```python
from build123d import *

# Parameters (mm, degrees)
SKETCH2_W            = 10
SKETCH2_H            = 14.768412439
BOSS_EXTRUDE1_DEPTH  = 5
BOSS_EXTRUDE4_DEPTH  = 10
SKETCH9_W            = 10
SKETCH9_H            = 3.18
SKETCH9_H_2          = 3.888412439
CUT_EXTRUDE3_DEPTH   = 5
BOSS_EXTRUDE5_DEPTH  = 7.7
SKETCH12_R           = 0.75
BOSS_EXTRUDE7_DEPTH  = 2.75
FILLET1_R            = 2.5
SKETCH13_W           = 17.887250462
SKETCH13_H           = 46.229219396
CUT_EXTRUDE4_DEPTH   = 20
SKETCH15_W           = 10
SKETCH15_H           = 7.7
BOSS_EXTRUDE9_DEPTH  = 100
CUT_EXTRUDE5_DEPTH   = 100
SKETCH17_W           = 2.538779858
SKETCH17_H           = 107.754476916
BOSS_EXTRUDE10_DEPTH = 5
FILLET2_R            = 3
FILLET3_R            = 3


with BuildPart() as part:
    # Sketch2 → Boss-Extrude1 (new body)
    with BuildSketch(Plane.XY):
        with Locations((0, 1.566049366)):
            Rectangle(SKETCH2_W, SKETCH2_H)
    extrude(amount=BOSS_EXTRUDE1_DEPTH)

    # Sketch8 → Boss-Extrude4 (add)
    with BuildSketch(Plane.ZY.offset(5)):
        Polygon((-0.15, 5.770255585), (0, 5.770255585), (0, 4.070255585), (-0.15, 4.070255585), (-2.137867966, 4.070255585), (-3.402081528, 5.334469147), (-2.2, 6.536550675), (-1.43370491, 5.770255585), align=None)
        Polygon((-0.15, -1.929744415), (0, -1.929744415), (0, -0.229744415), (-0.15, -0.229744415), (-1.43370491, -0.229744415), (-2.2, 0.536550675), (-3.402081528, -0.665530853), (-2.137867966, -1.929744415), align=None)
    extrude(amount=-BOSS_EXTRUDE4_DEPTH)

    # Sketch9 → Cut-Extrude3 (cut)
    with BuildSketch(Plane(origin=(0, 0, 0), x_dir=(-1, 0, 0), z_dir=(0, 0, -1))):
        with Locations((0, 7.360255585)):
            Rectangle(SKETCH9_W, SKETCH9_H)
        with Locations((0, -3.873950635)):
            Rectangle(SKETCH9_W, SKETCH9_H_2)
    extrude(amount=-CUT_EXTRUDE3_DEPTH, mode=Mode.SUBTRACT)

    # Sketch10 → Boss-Extrude5 (add)
    with BuildSketch(Plane(origin=(0, 5.770255585, 0), x_dir=(1, 0, 0), z_dir=(0, 1, 0))):
        with BuildLine():
            Line((-5, -5), (-5, -10.5))
            Line((-5, -10.5), (1.352445729, -55.7))
            Line((1.352445729, -55.7), (6.352445729, -55.7))
            Line((6.352445729, -55.7), (6.352445729, -49.2))
            ThreePointArc((6.352445729, -49.2), (1.383429579, -31.764936646), (5, -14))
            Line((5, -14), (5, -5))
            Line((5, -5), (-5, -5))
        make_face()
    extrude(amount=-BOSS_EXTRUDE5_DEPTH)

    # Sketch12 → Boss-Extrude7 (add)
    with BuildSketch(Plane.XY):
        with BuildLine():
            Line((5, 5.770255585), (8.5, 5.770255585))
            ThreePointArc((8.5, 5.770255585), (12.35, 1.920255585), (8.5, -1.929744415))
            Line((8.5, -1.929744415), (5, -1.929744415))
            Line((5, -1.929744415), (5, 5.770255585))
        make_face()
        with Locations((8.5, 1.920255585)):
            Circle(SKETCH12_R, mode=Mode.SUBTRACT)
    extrude(amount=BOSS_EXTRUDE7_DEPTH)

    # Fillet1
    fillet1_edges = [part.edges().sort_by_distance(p)[0] for p in [
        (6.352445729, 1.920255585, 49.2),
        (5, 1.920255585, 14),
        (1.352445729, 1.920255585, 55.7),
        (6.352445729, 1.920255585, 55.7),
    ]]
    fillet(fillet1_edges, radius=FILLET1_R)

    # Sketch13 → Cut-Extrude4 (cut)
    with BuildSketch(Plane(origin=(0, 5.770255585, 0), x_dir=(1, 0, 0), z_dir=(0, 1, 0))):
        with Locations((3.943625231, -33.614609698)):
            Rectangle(SKETCH13_W, SKETCH13_H)
    extrude(amount=-CUT_EXTRUDE4_DEPTH, mode=Mode.SUBTRACT)

    # Sketch15 → Boss-Extrude9 (add)
    with BuildSketch(Plane.XY.offset(10.5)):
        with Locations((0, 1.920255585)):
            Rectangle(SKETCH15_W, SKETCH15_H)
    extrude(amount=BOSS_EXTRUDE9_DEPTH)

    # Sketch16 → Cut-Extrude5 (cut)
    with BuildSketch(Plane(origin=(0, 5.770255585, 0), x_dir=(1, 0, 0), z_dir=(0, 1, 0))):
        Polygon((-5, -7.952810564), (2.461220142, -110.5), (-5, -110.5), align=None)
    extrude(amount=-CUT_EXTRUDE5_DEPTH, mode=Mode.SUBTRACT)

    # Sketch17 → Boss-Extrude10 (add)
    with BuildSketch(Plane(origin=(0, 5.770255585, 0), x_dir=(1, 0, 0), z_dir=(0, 1, 0))):
        with Locations((3.730610071, -56.622761542)):
            Rectangle(SKETCH17_W, SKETCH17_H)
    extrude(amount=BOSS_EXTRUDE10_DEPTH)

    # Fillet2
    fillet2_edges = [part.edges().sort_by_distance(p)[0] for p in [
        (2.461220142, 5.770255585, 56.622761542),
    ]]
    fillet(fillet2_edges, radius=FILLET2_R)

    # Fillet3
    # the kernel refuses this fillet: 3 mm, written as the material it takes off along each edge
    with BuildSketch(Plane(origin=(2.461220142, 10.770255585, 116.846949644), x_dir=(-0.016047608738208652, -0.9998712288358863, 0), z_dir=(0, 0, -1))) as fillet3_piece_1:
        with BuildLine():
            CenterArc((2.92841725, -2.967518469), FILLET3_R, 98.438939572, 73.338315122)
            Line((-0.040741346, -2.538452936), (-0.337657205, -2.495546383))
            ThreePointArc((-0.337657205, -2.495546383), (-0.320332042, -1.264412185), (-0.299961369, 0.004814283))
            Line((-0.299961369, 0.004814283), (0.004814283, 0.299961369))
            ThreePointArc((0.004814283, 0.299961369), (2.00455674, 0.267866151), (2.444124669, 0.296751847))
            Line((2.444124669, 0.296751847), (2.488151267, 0))
        make_face()
    extrude(amount=120.448376205, mode=Mode.SUBTRACT)


solid = part.part
```
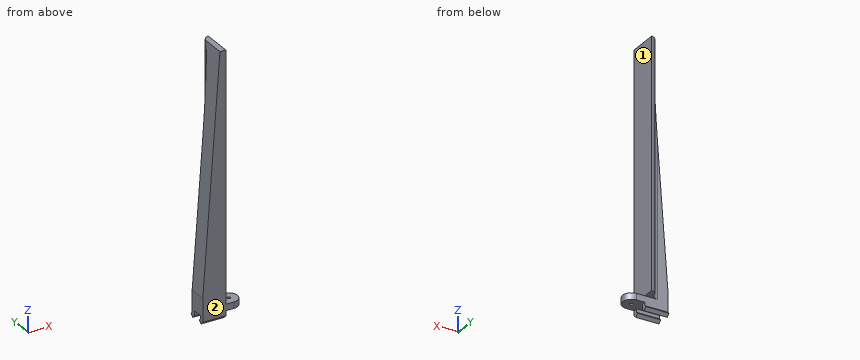
Work out the finished part from the listing and answer in its coordinate system (mm). Face numbers are marked on the shaded views. A direction names the side the tool comes from. Round coordinates to 2 decimals unless told otherwise and drop trailing zeros. Write each loop counter-clockwise with the first axis right and the second up, starting at its lowest first coordinate (ties: lowest second). Pieces come first, ordered by that corner, then holes. Notation, with made-up numbers: (22, 67) - (74, 67) arc R16 cw to (74, 86) - close; hole circle Ø3 at (39.25, 25). An arc over 180 degrees is marked (long way). Return JSON: item names as keys, results as strings. Group by question number.
Q1. The part is cut by section B-B on z = 38. Write down the section's boundary in (x, y), then the cut area to 3 significant figures.
Q2. For the marked faces 1 and 2, determine the directions among +Z, -Z, +X, -X, +Y, -Y from which every point of the face is accessible in a straight line to the end or side of a thin tool.
Q3. Each of these flat-tipped pins is pushed along its axis until it touches: pin 1 Ø1.2 at (y, z) = (5, -2) entering from +X; pin 2 Ø5 at (x, y) = (-2.5, 6) entering from -Z; pin 3 Ø0.7 at (x, z) = (-2.5, -1) entering from +Y; pin 4 Ø0.9 at (x, y) = (8.5, 1.92) entering from +Z. Where does it stop, or does it pass through?
Q4. Find the intervals of material crossed by L1, parallel to Y at x = 8.5, z = 0.7; L2, parallel to Y at x = -0.25, z = 8.5; L3, parallel to X at y = 1.5, z = 50, in increasing order.
Q5. The part is cut by section A-A on z = 66. Write down the section's boundary in (x, y), then the cut area to 3 significant figures.
Q6. The part is cut by section C-C on z = 85. Write down the section's boundary in (x, y).
Solved:
{
 "1": {"outline": "(-2.81, -1.93) - (5, -1.93) - (5, 10.77) arc R3 ccw to (2.42, 8.28) arc R3 cw to (-0.54, 5.77) - (-2.81, 5.77) - close", "area": "73.1 mm²"},
 "2": {"face 1": "+Z, +X, +Y, -Y", "face 2": "+Z, -Z, +X, -X, -Y"},
 "3": {"pin 1": "x = 5", "pin 2": "z = -3.4", "pin 3": "y = 5.77", "pin 4": "through"},
 "4": {"L1": "-1.93 to 1.17, 2.67 to 5.77", "L2": "-1.93 to 5.78", "L3": "-1.94 to 5"},
 "5": {"outline": "(-0.78, -1.93) - (5, -1.93) - (5, 10.77) arc R3 ccw to (2.42, 8.28) arc R3 cw to (-0.54, 5.77) - (-0.78, 5.77) - close", "area": "57.4 mm²"},
 "6": {"outline": "(0.61, -1.93) - (5, -1.93) - (5, 10.77) arc R3 ccw to (2.42, 8.28) arc R3 cw to (0.61, 6) - close"}
}
